from build123d import *

# Parameters (mm, degrees)
F0_W     = 25
F0_H     = 10
F3_D     = 25.1
F3_DEPTH = 200
F3_TIP   = 7.5408007688
F4_R     = 1
F5_SIZE  = 8
F6_R     = 1


with BuildPart() as f1:
    # F0 (on Top) → F1 (revolve)
    with BuildSketch(Plane.XY):
        with Locations((27.5, 62.9193106468)):
            Rectangle(F0_W, F0_H)
        Polygon((0, 87.9193106468), (0, -132.0806893532), (15, -132.0806893532), (15, 57.9193106468), (15, 67.9193106468), (40, 67.9193106468), (50, 67.9193106468), (50, 87.9193106468), align=None)
    revolve(axis=Axis((0, -22.0806893532, 0), (0, -1, 0)))

    # F3
    with Locations(Plane(origin=(0, 87.9193106468, 0), x_dir=(-1, 0, 0), z_dir=(0, 1, 0))):
        with Locations((0, 0)):
            Hole(F3_D / 2, depth=F3_DEPTH)
            with Locations((0, 0, -(F3_DEPTH + F3_TIP / 2))):  # 118° drill point
                Cone(0, F3_D / 2, F3_TIP, mode=Mode.SUBTRACT)

    # F4
    f4_edges = [f1.edges().sort_by_distance(p)[0] for p in [
        (-50, 87.919311, 0),
        (-15, -132.080689, 0),
    ]]
    fillet(f4_edges, radius=F4_R)

    # F5
    f5_edges = [f1.edges().sort_by_distance(p)[0] for p in [
        (-40, 57.919311, 0),
    ]]
    chamfer(f5_edges, length=F5_SIZE)

    # F6
    f6_edges = [f1.edges().sort_by_distance(p)[0] for p in [
        (-50, 67.919311, 0),
    ]]
    fillet(f6_edges, radius=F6_R)


solid = f1.part
Can you work these out from the model? Positions are in its coordinate system, mm. A direction names the side the tool comes from. Round coordinates to 2 decimals unless told otherwise and drop trailing zeros. Write each loop counter-clockwise with the first axis right and the second up, starting at its lowest first coordinate (ties: lowest second). Pieces come first, ordered by that corner, then holes. Notation, with made-up numbers: M 89,-30.5 L 104,-30.5 A22 ccw 104,6.5 Z; hole C -12.5,37 d10. An arc over 180 degrees is marked long. Use a Markdown table: item, result.
Item 1: We'd pull the mould along Z, two halves only. Please class faces 4 (the face through (10, 87.919, -10)), 5 (the face through (0.47, -118.31, -2.13)), 6 (the face through (-14.985, -35.258, 0.66)): released by +Z, released by -Z, zero draft, split by the parting line, or undercut.
Found:
| item | result |
|---|---|
| face 4 | zero draft |
| face 5 | undercut |
| face 6 | split by the parting line |
Item 2: I want a section at A-A (y = -6). List the corners of the cut face in (x, z) for me, and give its area (3 significant figures).
Found:
| item | result |
|---|---|
| outline | C 0,0 d30; hole C 0,0 d25.1 |
| area | 212 mm2 |
Item 3: Which directions (+Z, -Z, +X, -X, +Y, -Y) give clear straight access to the entire face, cutting with the end or side of a thin tool? Please do faces 1 (the face through (11.59, -13.48, -4.81)), 2 (the face through (-8.67, 66.93, -39.05)), 3 (the face through (0, -132.081, 0)).
Found:
| item | result |
|---|---|
| face 1 | +Y |
| face 2 | -Y |
| face 3 | +Z, -Z, +X, -X, -Y |
Item 4: If I drill on line 1 along Z through (x, y) = (0, -32.5); line 2 along Y through (x, z) = (31.5, -28); line 3 along X through (y, z) = (-100.5, -8), over which ranges is the centre line in solid material (lowest first)? Write a range as [from, to].
Found:
| item | result |
|---|---|
| line 1 | z = [-15, -12.55], [12.55, 15] |
| line 2 | y = [67.92, 87.92] |
| line 3 | x = [-12.69, -9.67], [9.67, 12.69] |
Item 5: For pin 1 Ø6 at (x, z) = (33.5, 12) entering from -Y; pin 2 Ø12 at (y, z) = (17.5, -2) entering from -X, each with a flat end and sliding along its axis, tell me the tip position at first contact or that it passes through.
Found:
| item | result |
|---|---|
| pin 1 | stops at y = 58.5 |
| pin 2 | stops at x = -15 |
